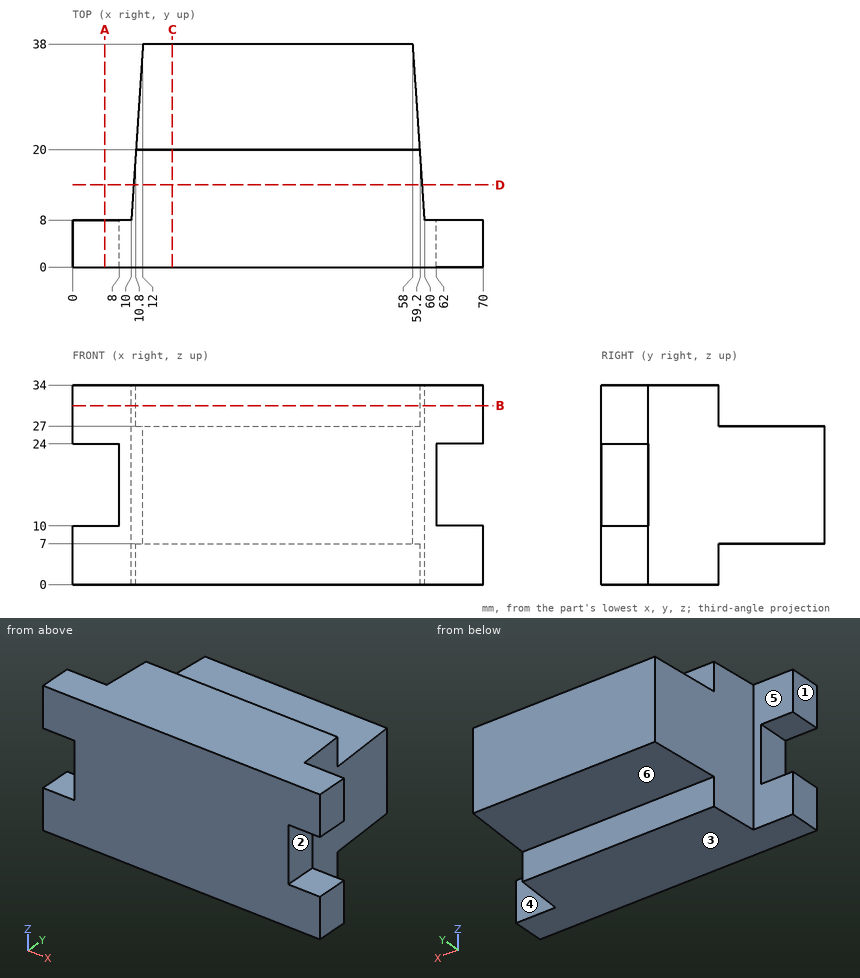
Geometry check sheet. Reference: drawing and pictorial views, mm from the part's lowest x, y, z. A direction names the side the tool comes from. Round coordinates to 2 decimals unless told otherwise and drop trailing zeros. Loops run counter-clockwise (first coordinate to the right, second up) from the corner with the lowest first, then second, coordinate; pieces in that order, holes last. Notation, with made-up numbers: M -3,-24 L 43,-24 A28 ccw 43,-2 Z; hole C 2,-11 d10. An arc over 180 degrees is marked long. Return JSON: item names as keys, results as strings. Group by question number.
(1) Scan lines: line 1 along X through (y, z) = (3, 23); line 2 along Z through (x, y) = (32.5, 34); line 3 along Y through (x, z) = (6, 5). Record each from-to range of solid material in increasing order. Write a range as [from, to].
(2) Section check C-C, the plane x = 17. Enter the section's corners in (y, z).
(3) Section check A-A, the plane x = 5.5. Enter the section's corners in (y, z), and give its area (3 significant figures).
(4) Section check D-D, the plane y = 14. Enter the section's corners in (x, z).
(5) Set-up check for the marked faces 4, 5 and 6: record each of +Z, -Z, +X, -X, +Y, -Y from which the full face is reachable in a straight line by a thin tool's end or side.
(6) Section check B-B, the plane z = 30.5. Enter the section's corners in (x, y), and give its area (3 significant figures).
(7) Mould release check, pull along Z, two halves, no side actions. Record for the marked faces 1, 2 and 3: pulls with the +Z half, pulls with the -Z half, needs draft (parallel to the pull), parting line crosses it, or undercut.
(8) Go/stop test with flat-tipped pins: pin 1 (2 mm diameter, centred on x = 31, z = 5, fed in from +Y); pin 2 (12 mm diameter, centred on y = 29.5, z = 21.5, fed in from -X); pin 3 (1.5 mm diameter, centred on y = 12, z = 23, fed in from +X). Record where each tip stops, or that it passes through.
Data:
{
 "1": {"line 1": "[8, 62]", "line 2": "[7, 27]", "line 3": "[0, 8]"},
 "2": {"outline": "M 0,0 L 20,0 L 20,7 L 38,7 L 38,27 L 20,27 L 20,34 L 0,34 Z"},
 "3": {"outline": "M 0,0 L 8,0 L 8,10 L 0,10 Z; M 0,24 L 8,24 L 8,34 L 0,34 Z", "area": "160 mm²"},
 "4": {"outline": "M 10.4,0 L 59.6,0 L 59.6,34 L 10.4,34 Z"},
 "5": {"face 4": "+Z, -Z, +X, +Y", "face 5": "+Z, -Z, -X, +Y", "face 6": "-Z, +X, -X, +Y"},
 "6": {"outline": "M 0,0 L 70,0 L 70,8 L 60,8 L 59.2,20 L 10.8,20 L 10,8 L 0,8 Z", "area": "1,150 mm²"},
 "7": {"face 1": "needs draft", "face 2": "undercut", "face 3": "pulls with the -Z half"},
 "8": {"pin 1": "y = 20", "pin 2": "x = 11.03", "pin 3": "x = 59.78"}
}
